from build123d import *

# Parameters (mm, degrees)
EXTRUDE_1_DEPTH     = 1.24
CUT_EXTRUDE_1_DEPTH = 1.24
SKETCH_4_W          = 8.4
SKETCH_4_H          = 3
EXTRUDE_2_DEPTH     = 2.2
CHAMFER_1_SIZE      = 1.2
CHAMFER_1_SIZE_2    = 2.4


with BuildPart() as part:
    # Эскиз1 → Бобышка-Вытянуть1 (new body)
    with BuildSketch(Plane.XY):
        with BuildLine():
            Line((-4.6, 0), (-4.6, 6.174949393))
            ThreePointArc((-4.6, 6.174949393), (-6.88149693, 3.454706934), (-7.7, 0))
            Line((-7.7, 0), (-7.7, -20.6))
            Line((-7.7, -20.6), (7.7, -20.6))
            Line((7.7, -20.6), (7.7, 0))
            ThreePointArc((7.7, 0), (6.88149693, 3.454706934), (4.6, 6.174949393))
            Line((4.6, 6.174949393), (4.6, 0))
            ThreePointArc((4.6, 0), (0, -4.6), (-4.6, 0))
        make_face()
    extrude(amount=EXTRUDE_1_DEPTH)

    # Эскиз3 → Вырез-Вытянуть1 (cut)
    with BuildSketch(Plane.XY.offset(1.24)):
        with BuildLine():
            Line((-7.7, -20.6), (-4.2, -20.6))
            Line((-4.2, -20.6), (-4.2, -15.2))
            ThreePointArc((-4.2, -15.2), (-5.1372583, -12.9372583), (-7.4, -12))
            Line((-7.4, -12), (-7.7, -12))
            Line((-7.7, -12), (-7.7, -20.6))
        make_face()
        with BuildLine():
            Line((4.2, -20.6), (4.2, -15.2))
            ThreePointArc((4.2, -15.2), (5.1372583, -12.9372583), (7.4, -12))
            Line((7.4, -12), (7.7, -12))
            Line((7.7, -12), (7.7, -20.6))
            Line((7.7, -20.6), (4.2, -20.6))
        make_face()
    extrude(amount=-CUT_EXTRUDE_1_DEPTH, mode=Mode.SUBTRACT)

    # Эскиз4 → Бобышка-Вытянуть2 (add)
    with BuildSketch(Plane.XY.offset(1.24)):
        with Locations((0, -19.1)):
            Rectangle(SKETCH_4_W, SKETCH_4_H)
    extrude(amount=EXTRUDE_2_DEPTH)

    # Фаска1
    # the kernel refuses this chamfer: 2.4, 1.2 mm, written as the material it adds along each edge
    with BuildSketch(Plane(origin=(4.2, -17.6, 1.24), x_dir=(0, 0.9976223042390325, -0.06891834360170876), z_dir=(-1, 0, 0))) as chamfer_1_piece_1_section:
        Polygon((CHAMFER_1_SIZE * 0.997622304239, -CHAMFER_1_SIZE * 0.0689183436017), (-CHAMFER_1_SIZE_2 * 0.0689183436017, -CHAMFER_1_SIZE_2 * 0.997622304239), (0, 0), align=None)
    chamfer_1_piece_1 = extrude(amount=8.4, mode=Mode.PRIVATE)
    chamfer_1_piece_1 = split(chamfer_1_piece_1, bisect_by=Plane(origin=(0, -17.211387721, 3.44), z_dir=(0, 0, -1)), keep=Keep.TOP, mode=Mode.PRIVATE)
    add(chamfer_1_piece_1)


solid = part.part
Source: CAD feature listing. Evaluate the final solid. Frame: model axes, mm. A direction names the side the tool comes from. Give positions to 0.01 mm unless a question says otherwise; leave off trailing zeros. Order: outer loops, then holes, each group sorted by start corner. A loop starts at its lowest first (then second) coordinate and runs counter-clockwise, first axis right, second up. Notation, with made-up numbers: (12.25, -3.75) -> (37.25, -3.75) arc R20 ccw to (37.25, 14.25) -> close; hole circle Ø1 at (23, 81.25). An arc over 180 degrees is marked (long way). Use a Markdown table: item, result.
1) Reachability of faces 5 (the cylindrical face through (6.904, 3.41, 0.611)), 6 (the flat face through (4.6, 3, 1)), 7 (the flat face through (0, -7, 0)), 8 (the flat face through (0, -7, 1.24)), 9 (the flat face through (4.2, -18, 2)) from +Z, -Z, +X, -X, +Y, -Y: full face, straight path, thin tool, end or side. Return the list, or none.
Answer list:
| item | result |
|---|---|
| face 5 | +Z, -Z, +X, +Y |
| face 6 | +Z, -Z, +Y |
| face 7 | -Z, +X, -X, +Y, -Y |
| face 8 | +Z, +X, -X, +Y |
| face 9 | +Z, -Z, +X, -Y |
2) Section query A-A, the plane y = 1. Return the cut outline in (x, z), then the cut area to 3 significant figures.
Answer list:
| item | result |
|---|---|
| outline | (-7.63, 0) -> (-4.6, 0) -> (-4.6, 1.24) -> (-7.63, 1.24) -> close; (4.6, 0) -> (7.63, 0) -> (7.63, 1.24) -> (4.6, 1.24) -> close |
| area | 7.53 mm² |
3) Section query B-B, the plane x = 0. Return the cut outline in (y, z), then the cut area to 3 significant figures.
Answer list:
| item | result |
|---|---|
| outline | (-20.6, 0) -> (-4.6, 0) -> (-4.6, 1.24) -> (-16.4, 1.24) -> (-17.5, 3.44) -> (-20.6, 3.44) -> close |
| area | 27.9 mm² |
4) Section query D-D, the plane z = 1.7. Return the cut outline in (x, y).
Answer list:
| item | result |
|---|---|
| outline | (-4.2, -20.6) -> (4.2, -20.6) -> (4.2, -16.63) -> (-4.2, -16.63) -> close |
5) Mould query, pull axis X, two halves, no side actions, for faces 1 (the flat face through (-4.2, -18, 2)), 2 (the cylindrical face through (0.1, -4.6, 0.6)), 3 (the cylindrical face through (5.113, -12.962, 0.629)), 4 (the flat face through (0, -20.6, 2)). Classes: +X half, -X half, draft (parallel to the pull), parting line (faces both ways), or undercut.
Answer list:
| item | result |
|---|---|
| face 1 | -X half |
| face 2 | undercut |
| face 3 | +X half |
| face 4 | draft |
6) Ray query, line 1 along Z through (x, y) = (6.5, -5.25); line 2 along X through (y, z) = (-15.5, 0.3); line 3 along X through (y, z) = (-3.75, 1.1). Return the intervals inside material, ascending. Write a range as [from, to].
Answer list:
| item | result |
|---|---|
| line 1 | [0, 1.24] |
| line 2 | [-4.2, 4.2] |
| line 3 | [-7.7, -2.66], [2.66, 7.7] |
7) Section query C-C, the plane y = -15.5. Return the cut outline in (x, z).
Answer list:
| item | result |
|---|---|
| outline | (-4.2, 0) -> (4.2, 0) -> (4.2, 1.24) -> (-4.2, 1.24) -> close |
8) Contact query for flat-ended pins moving along their axis: P1, Ø1, axis at y = 4.5, z = 0.5, coming from the +X side; P2, Ø1.5, axis at y = -17, z = 0.5, coming from the +X side; P3, Ø0.6, axis at y = 2, z = 1, coming from the -X side; P4, Ø2, axis at x = -6, z = 2.5, coming from the -Y side. Output: stop coordinate, or through.
Answer list:
| item | result |
|---|---|
| P1 | x = 6.58 |
| P2 | x = 4.2 |
| P3 | x = -7.51 |
| P4 | through |
